Geometry check sheet. Reference: the model listing, model coordinates, mm. A direction names the side the tool comes from. Give positions to 0.01 mm unless a question says otherwise; leave off trailing zeros. Order: outer loops, then holes, each group sorted by start corner. A loop starts at its lowest first (then second) coordinate and runs counter-clockwise, first axis right, second up. Notation, with made-up numbers: M 8.5,48.5 L 36.5,48.5 A14 cw 36.5,73.5 Z; hole C 55,17 d2. An arc over 180 degrees is marked long. Put each result on its own line as item: value. Start each with the question number.
Q1. Section check D-D on z = -51.87. Record the cut outline in (x, y).
Q2. Access from +Z, -Z, +X, -X, +Y, -Y to the whole of each face (thin tool, end or side, straight path). Record for faces 5 (the flat face through (-56, 7.5, -36)), 6 (the flat face through (-21, 40, -24)).
Q3. Section check C-C on y = 2. Record the cut outline in (x, z), then the cut area to 3 significant figures.
Q4. Section check B-B on y = 21.5. Record the cut outline in (x, z).
Q5. Mould release check, pull along X, two halves, no side actions. Record for faces 1 (the cylindrical face through (-63.01, 3.698, -48.175)), 2 (the cylindrical face through (-58.053, 36.198, -27.867)), 3 (the flat face through (-62.463, 3.698, -26.919)), 4 (the cylindrical face through (-66.798, 36.198, -57.845)): +X half, -X half, draft (parallel to the pull), parting line (faces both ways), or undercut.
Q6. Material ranges on L1, parallel to Z at x = -26, y = 11; L2, parallel to Z at x = 14.5, y = 5.5, recorded low to high.
Q7. Section check A-A on z = -27. Record the cut outline in (x, y), then the cut area to 3 significant figures.
Q8. Go/stop test with flat-tipped pins: pin 1 (10 mm diameter, centred on x = 36.5, y = 12.5, fed in from -Z); pin 2 (4 mm diameter, centred on y = 8.5, z = -13, fed in from +X); pin 3 (8 mm diameter, centred on x = 14, y = 5, fed in from -Z). Record where each tip stops, or that it passes through.
```python
from build123d import *

# Parameters (mm, degrees)
SKETCH1_R           = 4
BOSS_EXTRUDE1_DEPTH = 40
SKETCH2_W           = 23
SKETCH2_H           = 25
CUT_EXTRUDE1_DEPTH  = 101.058107917


with BuildPart() as part:
    # Sketch1 → Boss-Extrude1 (new body)
    with BuildSketch(Plane(origin=(0, 0, 0), x_dir=(1, 0, 0), z_dir=(0, 1, 0))):
        with BuildLine():
            Line((39.60733846, 0), (52.847209838, 0))
            ThreePointArc((52.847209838, 0), (56.811389388, 1.952824177), (57.67903067, 6.285887802))
            Line((57.67903067, 6.285887802), (56.02903067, 12.485887802))
            ThreePointArc((56.02903067, 12.485887802), (54.923989844, 14.533333284), (53.012004514, 15.85902568))
            Line((53.012004514, 15.85902568), (-58.57444061, 59.324441087))
            ThreePointArc((-58.57444061, 59.324441087), (-66.890236963, 57.761426345), (-69.151600504, 49.607794087))
            Line((-69.151600504, 49.607794087), (-55.584042349, 3.586121305))
            ThreePointArc((-55.584042349, 3.586121305), (-53.782323718, 0.995665256), (-50.788112092, 0))
            Line((-50.788112092, 0), (-22.483562644, 0))
            ThreePointArc((-22.483562644, 0), (8.561887908, 13.48), (39.60733846, 0))
        make_face()
        with Locations(Location((-61.478112092, 51.87, 0), (0, 0, 270))):
            Circle(SKETCH1_R, mode=Mode.SUBTRACT)
        with Locations(Location((-54.148112092, 27, 0), (0, 0, 270))):
            Circle(SKETCH1_R, mode=Mode.SUBTRACT)
    extrude(amount=BOSS_EXTRUDE1_DEPTH)

    # Sketch2 → Cut-Extrude1 (cut, through all)
    with BuildSketch(Plane.XY):
        with Locations((-57.978112092, 20)):
            Rectangle(SKETCH2_W, SKETCH2_H)
    extrude(amount=-CUT_EXTRUDE1_DEPTH, mode=Mode.SUBTRACT)


solid = part.part
```
Results found:
1. outline: M -69.48,0 L -65.48,0 L -65.48,7.5 L -69.48,7.5 Z; M -69.48,32.5 L -65.48,32.5 L -65.48,40 L -69.48,40 Z; M -57.48,0 L -39.44,0 L -39.44,40 L -57.48,40 L -57.48,32.5 L -46.48,32.5 L -46.48,7.5 L -57.48,7.5 Z
2. face 5: +Z, -Z, -X
2. face 6: +Z, -Z, +X, -X, +Y
3. outline: M -69.15,-49.61 A8 ccw -58.57,-59.32 L 53.01,-15.86 A5 ccw 56.03,-12.49 L 57.68,-6.29 A5 ccw 52.85,0 L 39.61,0 A42.49 cw -22.48,0 L -50.79,0 A5 ccw -55.58,-3.59 Z; hole C -61.48,-51.87 d8; hole C -54.15,-27 d8
3. area: 3,830 mm^2
4. outline: M -46.48,-54.61 L 53.01,-15.86 A5 ccw 56.03,-12.49 L 57.68,-6.29 A5 ccw 52.85,0 L 39.61,0 A42.49 cw -22.48,0 L -46.48,0 Z
5. face 1: undercut
5. face 2: undercut
5. face 3: -X half
5. face 4: parting line
6. L1: z = -46.64 to 0
6. L2: z = -30.86 to -13.06
7. outline: M -62.49,0 L -58.15,0 L -58.15,7.5 L -62.49,7.5 Z; M -62.49,32.5 L -58.15,32.5 L -58.15,40 L -62.49,40 Z; M -50.15,0 L 24.41,0 L 24.41,40 L -50.15,40 L -50.15,32.5 L -46.48,32.5 L -46.48,7.5 L -50.15,7.5 Z
7. area: 2,960 mm^2
8. pin 1: stops at z = -24.24
8. pin 2: stops at x = 56.42
8. pin 3: stops at z = -32.61
